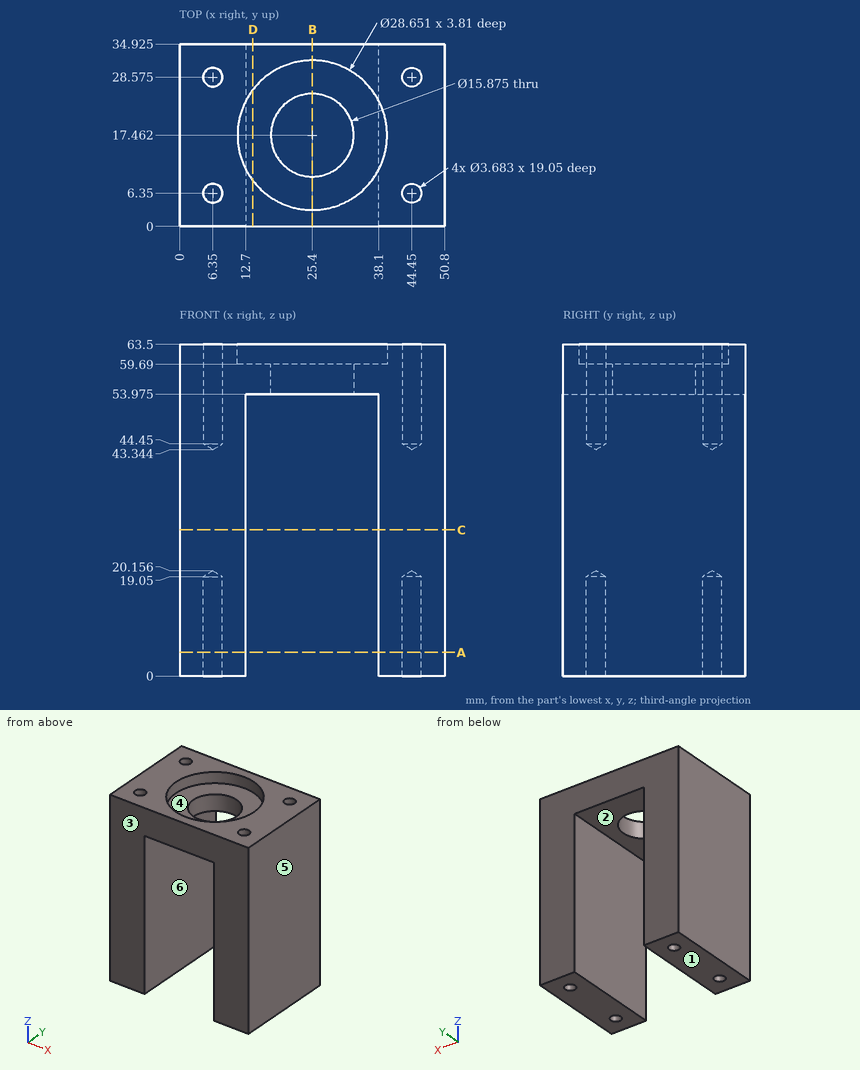
Input: dimensioned drawing with shaded views. Units: mm. Origin: part minimum x, y, z. A direction names the side the tool comes from. Round coordinates to 2 decimals unless told otherwise and drop trailing zeros. Write each loop counter-clockwise with the first axis right and the second up, starting at its lowest first coordinate (ties: lowest second). Pieces come first, ordered by that corner, then holes. Notation, with made-up numbers: (77.25, 71) - (105.25, 71) arc R18 cw to (105.25, 79) - close; hole circle Ø3 at (85.5, 47). An arc over 180 degrees is marked (long way). Write item = value, one per line.
(1) Material intervals for probe 1 along Y at (x, z) = (6.35, 4.5) (1 decimal); probe 2 along X at (y, z) = (6.35, 9.25); probe 3 along X at (y, z) = (23.5, 20), sorted ascending.
Geometry check:
probe_1 = 0 to 4.5, 8.2 to 26.7, 30.4 to 34.9
probe_2 = 0 to 4.51, 8.19 to 12.7, 38.1 to 42.61, 46.29 to 50.8
probe_3 = 0 to 12.7, 38.1 to 50.8
(2) Section query B-B on x = 25.4. Output: boundary loops of the cut face in (y, z) (1 decimal).
Geometry check:
outline = (0, 54) - (9.5, 54) - (9.5, 59.7) - (3.1, 59.7) - (3.1, 63.5) - (0, 63.5) - close; (25.4, 54) - (34.9, 54) - (34.9, 63.5) - (31.8, 63.5) - (31.8, 59.7) - (25.4, 59.7) - close
(3) Pull-direction query (X, two-part tool) for the marked faces 3, 4, 5 and 6; classes: +X half, -X half, draft (parallel to the pull), parting line (faces both ways), or undercut.
Geometry check:
face_3 = draft
face_4 = undercut
face_5 = +X half
face_6 = undercut
(4) Section query C-C on z = 28. Output: boundary loops of the cut face in (x, y) (1 decimal).
Geometry check:
outline = (0, 0) - (12.7, 0) - (12.7, 34.9) - (0, 34.9) - close; (38.1, 0) - (50.8, 0) - (50.8, 34.9) - (38.1, 34.9) - close
(5) Access query for the marked faces 1 and 2. Directions: +Z, -Z, +X, -X, +Y, -Y. A direction counts if a zero-diameter tool reaches every point of the face in a straight line with its end or side. Return the directions, or none.
Geometry check:
face_1 = -Z, +X, -X, +Y, -Y
face_2 = -Z, +Y, -Y
(6) Contact query for flat-ended pins moving along their axis: pin 1 Ø1 at (x, y) = (21.5, 4.5) entering from -Z (1 decimal); pin 2 Ø2 at (x, y) = (44.45, 28.575) entering from +Z (1 decimal); pin 3 Ø17 at (x, y) = (25.4, 17.46) entering from +Z. Output: stop coordinate, or through.
Geometry check:
pin_1 = 54
pin_2 = 43.9
pin_3 = 59.69
(7) Section query A-A on z = 4.5. State how many separate pieces and enclosed holes the cut face has.
Geometry check:
separate_pieces = 2
enclosed_holes = 4
(8) Section query D-D on x = 14. Output: boundary loops of the cut face in (y, z) (1 decimal).
Geometry check:
outline = (0, 54) - (34.9, 54) - (34.9, 63.5) - (26.1, 63.5) - (26.1, 59.7) - (8.8, 59.7) - (8.8, 63.5) - (0, 63.5) - close
